Part print with two shaded views. Sizes in mm from the minimum x, y, z corner. A direction names the side the tool comes from. Round coordinates to 2 decimals unless told otherwise and drop trailing zeros. Write each loop counter-clockwise with the first axis right and the second up, starting at its lowest first coordinate (ties: lowest second). Pieces come first, ordered by that corner, then holes. Notation, with made-up numbers: M -19.75,76 L 11.25,76 A26 cw 11.25,93 Z; hole C 52,3.5 d6. An arc over 180 degrees is marked long. One line per question, with ' | ' between items. Start each with the question number.
1) Saw through at D-D (x = 260). List the corners of the cut face in (y, z), plus the area to 3 significant figures.
2) Saw through at B-B (x = 127.5). List the corners of the cut face in (y, z).
3) Wall check: probe 1 along X at (y, z) = (37, 244.5); probe 2 along Y at (x, z) = (226, 23.5); probe 3 along Y at (x, z) = (112.5, 139.5). Give the ranges that are in metal, low to high. Write a range as [from, to].
4) Tool access for the marked faces 1, 2 and 3: list every direction of +Z, -Z, +X, -X, +Y, -Y with a clear straight run to the whole face (end or side of a thin tool).
5) Saw through at A-A (z = 150). List the corners of the cut face in (x, y).
6) Drop flat-ended pins along their axis: pin 1 Ø1 at (x, y) = (156.5, 121) entering from -Z; pin 2 Ø1.8 at (x, y) = (52.5, 148.5) entering from +Z; pin 3 Ø8 at (y, z) = (117.5, 76) entering from +X. Give the stop position or say it passes through.
7) Saw through at C-C (y = 43). List the corners of the cut face in (x, z).
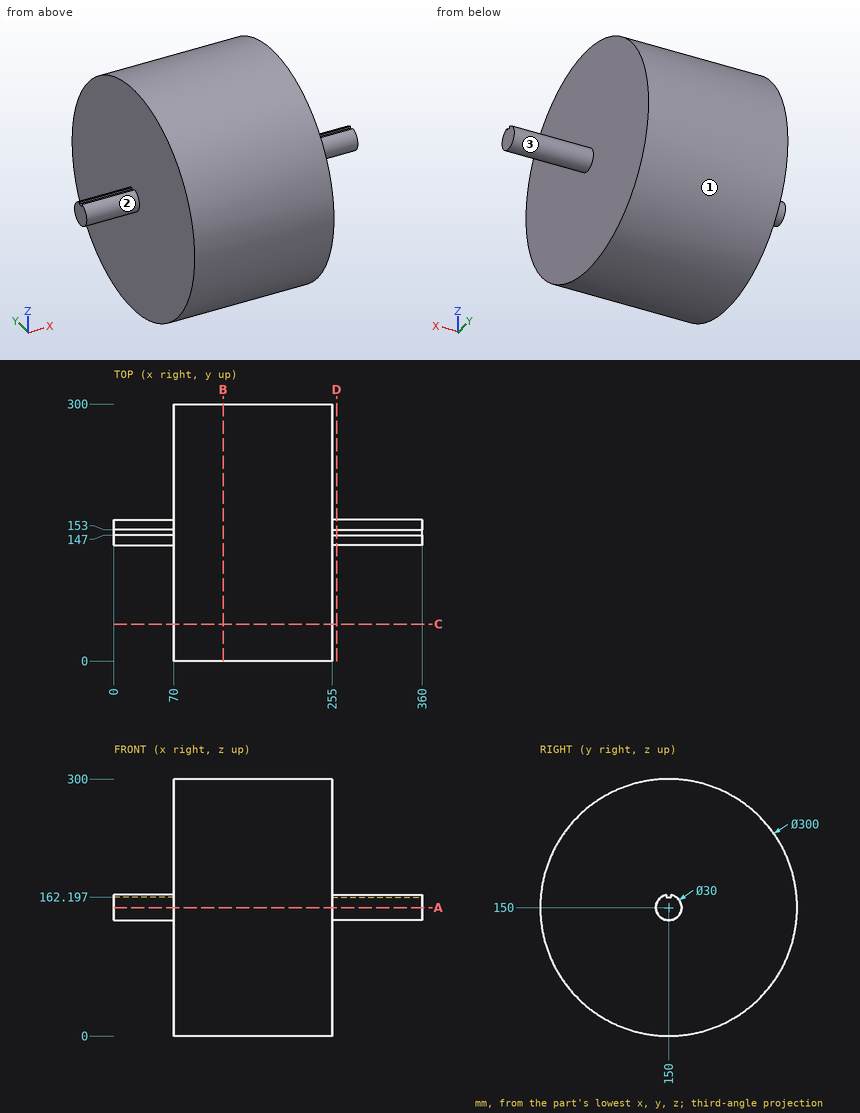
Answer key:
1) outline: M 147,162.2 L 147,164.7 A15 ccw long 153,164.7 L 153,162.2 Z | area: 691 mm2
2) outline: C 150,150 d300
3) probe 1: x = [70, 255] | probe 2: y = [69.39, 230.61] | probe 3: y = [0.37, 299.63]
4) face 1: +X, -X | face 2: -X | face 3: +X
5) outline: M 0,135 L 70,135 L 70,0 L 255,0 L 255,135 L 360,135 L 360,165 L 255,165 L 255,300 L 70,300 L 70,165 L 0,165 Z
6) pin 1: stops at z = 2.73 | pin 2: stops at z = 162.2 | pin 3: stops at x = 255
7) outline: M 70,44.88 L 255,44.88 L 255,255.12 L 70,255.12 Z
